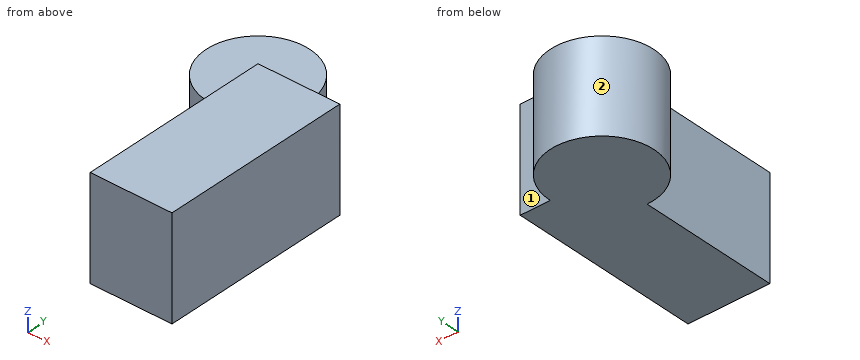
```python
from build123d import *

# Parameters (mm, degrees)
F0_R     = 28.0405076849
F1_DEPTH = 49.53
F2_W     = 44.3078614771
F2_H     = 55.0068765879
F3_DEPTH = 104.14


with BuildPart() as f1:
    # F0 (on Top) → F1 (new body)
    with BuildSketch(Plane.XY):
        Circle(F0_R)
    extrude(amount=F1_DEPTH)

    # F2 (on Front) → F3 (join)
    with BuildSketch(Plane.XZ):
        with Locations((22.1539307386, 27.5034382939)):
            Rectangle(F2_W, F2_H)
    extrude(amount=F3_DEPTH)


solid = f1.part
```
Design review of the part built by this model. Coordinates are the model's own, in mm. Face numbers are marked on the shaded views. A direction names the side the tool comes from. Coordinates: 2 decimals unless noted, no trailing zeros. Write each loop counter-clockwise with the first axis right and the second up, starting at its lowest first coordinate (ties: lowest second). Pieces come first, ordered by that corner, then holes.
1) To check wall thickness, follow L1, parallel to X at y = -50, z = 8; L2, parallel to Y at x = 38, z = 48; L3, parallel to Z at x = -6, y = -20. State the ranges of each line that lie inside material, in increasing order.
2) Add section B-B (y = -36). Write out the cut boundary in (x, z).
3) Add section C-C (x = 12). Write out the cut boundary in (y, z), plus the area to 3 significant figures.
4) Add section A-A (z = 13.5). Write out the cut boundary in (x, y), plus the area to 3 significant figures.
5) Add section D-D (y = -12). Write out the cut boundary in (x, z).
6) Insertion check: pin 1 (8 mm diameter, centred on y = -8, z = 10, fed in from -X); pin 2 (4 mm diameter, centred on x = -11, y = -28, fed in from -Z); pin 3 (10 mm diameter, centred on x = 11, z = 6.5, fed in from +Y); pin 4 (17 mm diameter, centred on x = -12, y = 2, fed in from +Z). Each pin has a flat end and moves straight along its axis. Give the tip position at first contact, or say it passes through.
7) Machinability: for the marked faces 1 and 2, which of the approach directions +Z, -Z, +X, -X, +Y, -Y give a long, thin tool a straight path to every point of the face, cutting with its end or side? Answer none if there is none.
Check result:
1. L1: x = 0 to 44.31
1. L2: y = -104.14 to 0
1. L3: z = 0 to 49.53
2. outline: (0, 0) - (44.31, 0) - (44.31, 55.01) - (0, 55.01) - close
3. outline: (-104.14, 0) - (25.34, 0) - (25.34, 49.53) - (0, 49.53) - (0, 55.01) - (-104.14, 55.01) - close
3. area: 6,980 mm2
4. outline: (0, -104.14) - (44.31, -104.14) - (44.31, 0) - (28.04, 0) arc R28.04 ccw (long way) to (0, -28.04) - close
4. area: 6,470 mm2
5. outline: (-25.34, 0) - (44.31, 0) - (44.31, 55.01) - (0, 55.01) - (0, 49.53) - (-25.34, 49.53) - close
6. pin 1: stops at x = -27.75
6. pin 2: passes through
6. pin 3: stops at y = 27.39
6. pin 4: stops at z = 49.53
7. face 1: +Z, +X, +Y
7. face 2: +Z, -Z
